```python
from build123d import *

# Parameters (mm, degrees)
F0_R     = 22.225
F1_DEPTH = 394.1064
F2_R     = 19.05
F3_DEPTH = 66.2686
F4_R     = 17.4625
F5_DEPTH = 53.848
F6_SIZE  = 1.5875
F9_DEPTH = 3.81


with BuildPart() as f1:
    # F0 (on Right) → F1 (new body)
    with BuildSketch(Plane.YZ):
        Circle(F0_R)
    extrude(amount=F1_DEPTH)

    # F2 (on face) → F3 (join)
    with BuildSketch(Plane.YZ.offset(394.1064)):
        Circle(F2_R)
    extrude(amount=F3_DEPTH)

    # F4 (on face) → F5 (join)
    with BuildSketch(Plane.YZ.offset(460.375)):
        Circle(F4_R)
    extrude(amount=F5_DEPTH)

    # F6
    f6_edges = [f1.edges().sort_by_distance(p)[0] for p in [
        (514.223, -17.4625, 0),
    ]]
    chamfer(f6_edges, length=F6_SIZE)

    # F8 (on offset) → F9 (cut)
    with BuildSketch(Plane.XY.offset(17.4625)):
        with BuildLine():
            Line((521.658003, 3.9624), (464.3374, 3.9624))
            ThreePointArc((464.3374, 3.9624), (460.375, 0), (464.3374, -3.9624))
            Line((464.3374, -3.9624), (521.658003, -3.9624))
            Line((521.658003, -3.9624), (521.658003, 3.9624))
        make_face()
    extrude(amount=-F9_DEPTH, mode=Mode.SUBTRACT)

    # F10: F1 across plane


with BuildPart() as f1_1:
    add(f1.part)
    add(f1.part.mirror(Plane.YZ))


solid = f1_1.part
```
Source: CAD feature listing. Evaluate the final solid. Frame: model axes, mm. A direction names the side the tool comes from. Coordinates: 2 decimals unless noted, no trailing zeros. Loops run counter-clockwise (first coordinate to the right, second up) from the corner with the lowest first, then second, coordinate; pieces in that order, holes last. Notation, with made-up numbers: M 85.5,-12 L 111.5,-12 A20 ccw 111.5,-7 Z; hole C 13,74 d1. An arc over 180 degrees is marked long. Put each result on its own line as item: value. Start each with the question number.
1) Reachability of faces 1 (the face through (460.375, 17, -6)), 2 (the face through (-394.106, 16.4, 10)), 3 (the face through (-514.223, 0, 0)) from +Z, -Z, +X, -X, +Y, -Y: full face, straight path, thin tool, end or side. Return the list, or none.
2) Cut plane B-B on x = -444. Return the cut outline in (y, z).
3) Contact query for flat-ended pins moving along their axis: pin 1 Ø2.5 at (x, y) = (494.5, 1) entering from +Z; pin 2 Ø10 at (x, y) = (-207, 15) entering from +Z; pin 3 Ø1 at (x, z) = (-493.5, 15.5) entering from -Y. Output: stop coordinate, or through.
4) Ray query, L1, parallel to Y at x = -223.5, z = 1.5; L2, parallel to Y at x = -189, z = -15.5; L3, parallel to Z at x = -309, y = -1. Return the intervals inside material, ascending. Write a range as from..to.
5) Cut plane A-A on x = -272.5. Return the cut outline in (y, z) (3 decimals), then the cut area to 3 significant figures.
The answers:
1. face 1: +X
1. face 2: -X
1. face 3: +Z, -Z, -X, +Y, -Y
2. outline: C 0,0 d38.1
3. pin 1: stops at z = 13.65
3. pin 2: stops at z = 19.85
3. pin 3: stops at y = -8.94
4. L1: y = -22.17..22.17
4. L2: y = -15.93..15.93
4. L3: z = -22.2..22.2
5. outline: C 0,0 d44.45
5. area: 1,550 mm²
